Study the drawing (mm; zero at the part's minimum x, y, z) and answer. Round coordinates to 2 decimals unless told otherwise and drop trailing zeros. Loops run counter-clockwise (first coordinate to the right, second up) from the corner with the lowest first, then second, coordinate; pieces in that order, holes last. Notation, with made-up numbers: M 61.5,-33 L 93.5,-33 A20 cw 93.5,4 Z; hole C -10,70 d10. An arc over 180 degrees is marked long. Put each result on its own line as item: value. Start each with the question number.
(1) Straight lines are drawn through the part: line 1 (Y direction, x = 13.5, z = 2); line 2 (Y direction, x = 67, z = 17). For each, find the intervals that lie inside material, in ascending order.
(2) Section B-B, the plane z = 17.75 is taken. Determine the outline of the cut face in (x, y), then the cut area to 3 significant figures.
(3) Section A-A, the plane x = 4 is taken. Determine the outline of the cut face in (y, z).
(4) Section C-C, the plane z = 1.25 is taken. Determine the outline of the cut face in (x, y).
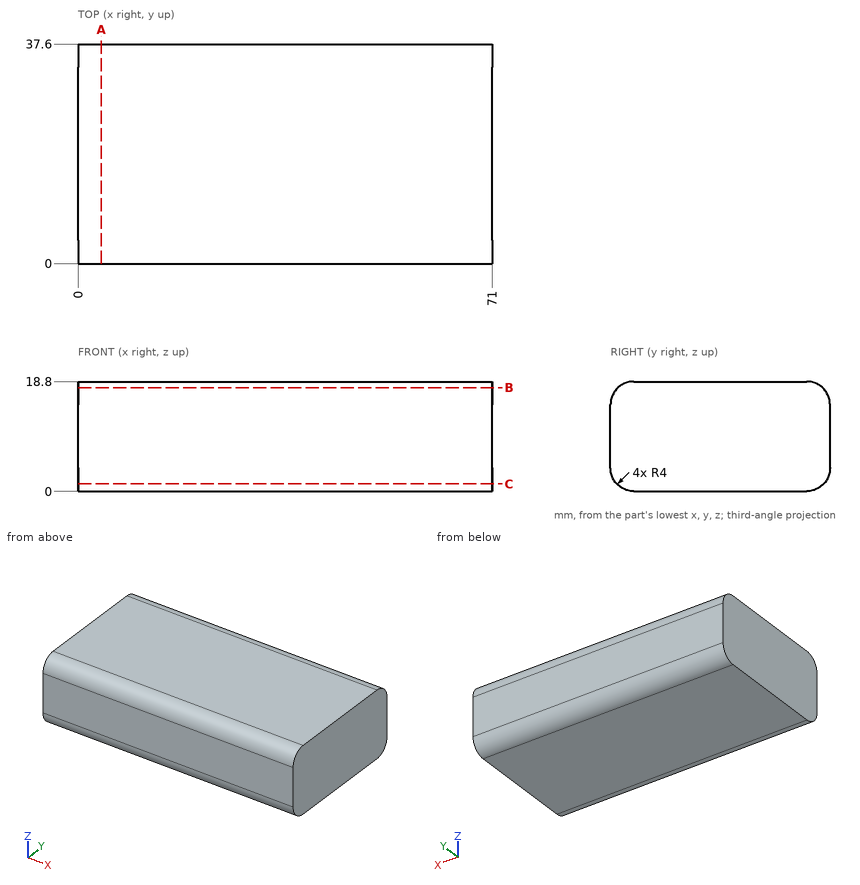
Recorded:
1. line 1: y = 0.54 to 37.06
1. line 2: y = 0.66 to 36.94
2. outline: M 0,1.3 L 71,1.3 L 71,36.3 L 0,36.3 Z
2. area: 2,490 mm²
3. outline: M 0,4 A4 ccw 4,0 L 33.6,0 A4 ccw 37.6,4 L 37.6,14.8 A4 ccw 33.6,18.8 L 4,18.8 A4 ccw 0,14.8 Z
4. outline: M 0,1.1 L 71,1.1 L 71,36.5 L 0,36.5 Z
